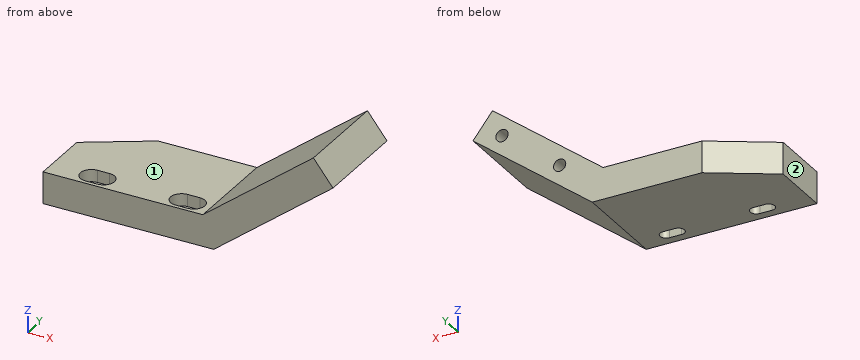
```python
from build123d import *

# Parameters (mm, degrees)
F1_DEPTH = 40
F3_DEPTH = 5
F5_DEPTH = 25
F7_DEPTH = 25
F8_R     = 2.5
F9_DEPTH = 15


with BuildPart() as f1:
    # F0 (on Front) → F1 (new body)
    with BuildSketch(Plane.XZ):
        Polygon((-70, 13), (-70, 0), (0, 0), (48.856667, 38.171011), (40.853068, 48.415151), (-4.476259, 13), align=None)
    extrude(amount=F1_DEPTH)

    # F2 (on face) → F3 (cut)
    with BuildSketch(Plane.XY.offset(13)):
        with BuildLine():
            Line((-16.5, -38.5), (-11.5, -38.5))
            ThreePointArc((-11.5, -38.5), (-7, -34), (-11.5, -29.5))
            Line((-11.5, -29.5), (-16.5, -29.5))
            ThreePointArc((-16.5, -29.5), (-21, -34), (-16.5, -38.5))
        make_face()
        with BuildLine():
            Line((-48.5, -29.5), (-53.5, -29.5))
            ThreePointArc((-53.5, -29.5), (-58, -34), (-53.5, -38.5))
            Line((-53.5, -38.5), (-48.5, -38.5))
            ThreePointArc((-48.5, -38.5), (-44, -34), (-48.5, -29.5))
        make_face()
    extrude(amount=-F3_DEPTH, mode=Mode.SUBTRACT)

    # F4 (on face) → F5 (cut)
    with BuildSketch(Plane.XY.offset(13)):
        with BuildLine():
            Line((-53.5, -36.5), (-48.5, -36.5))
            ThreePointArc((-48.5, -36.5), (-46, -34), (-48.5, -31.5))
            Line((-48.5, -31.5), (-53.5, -31.5))
            ThreePointArc((-53.5, -31.5), (-56, -34), (-53.5, -36.5))
        make_face()
        with BuildLine():
            Line((-11.5, -31.5), (-16.5, -31.5))
            ThreePointArc((-16.5, -31.5), (-19, -34), (-16.5, -36.5))
            Line((-16.5, -36.5), (-11.5, -36.5))
            ThreePointArc((-11.5, -36.5), (-9, -34), (-11.5, -31.5))
        make_face()
    extrude(amount=-F5_DEPTH, mode=Mode.SUBTRACT)

    # F6 (on face) → F7 (cut)
    with BuildSketch(Plane.XY.offset(13)):
        Polygon((-70, 0), (-70, -15), (-45, 0), align=None)
    extrude(amount=-F7_DEPTH, mode=Mode.SUBTRACT)

    # F8 (on face) → F9 (cut)
    with BuildSketch(Plane(origin=(0, 0, 0), x_dir=(-1, 0, 0), z_dir=(0, 1, 0))):
        with Locations((-36.97476, 37.136467)):
            Circle(F8_R)
        with Locations((-13.334437, 18.666622)):
            Circle(F8_R)
    extrude(amount=-F9_DEPTH, mode=Mode.SUBTRACT)


solid = f1.part
```
Geometry: final body of the model. Coordinates: model frame, mm. Face numbers are marked on the shaded views. A direction names the side the tool comes from. Round coordinates to 2 decimals unless told otherwise and drop trailing zeros. Write each loop counter-clockwise with the first axis right and the second up, starting at its lowest first coordinate (ties: lowest second). Pieces come first, ordered by that corner, then holes. Notation, with made-up numbers: (-29.75, 28) -> (-25.75, 28) arc R6 cw to (-25.75, 37) -> close; hole circle Ø10 at (74.5, 42). An arc over 180 degrees is marked (long way). Return JSON: item names as keys, results as strings.
Q1. Section A-A on y = -34. Return the cut outline in (x, z).
From the geometry:
{"outline": "(-70, 0) -> (-56, 0) -> (-56, 8) -> (-58, 8) -> (-58, 13) -> (-70, 13) -> close; (-46, 0) -> (-19, 0) -> (-19, 8) -> (-21, 8) -> (-21, 13) -> (-44, 13) -> (-44, 8) -> (-46, 8) -> close; (-9, 0) -> (0, 0) -> (48.86, 38.17) -> (40.85, 48.42) -> (-4.48, 13) -> (-7, 13) -> (-7, 8) -> (-9, 8) -> close"}
Q2. Ray query, line 1 (Z direction, x = -51, y = -23); line 2 (Y direction, x = -14, z = 5.5); line 3 (X direction, y = -10, z = 18). Return the intervals inside material, ascending.
From the geometry:
{"line 1": "0 to 13", "line 2": "-40 to -36.5, -31.5 to 0", "line 3": "1.92 to 10.92, 15.74 to 23.04"}
Q3. Section D-D on z = 30. Return the cut outline in (x, y), and give its area (3 significant figures).
From the geometry:
{"outline": "(17.28, -40) -> (38.4, -40) -> (38.4, 0) -> (17.28, 0) -> close", "area": "845 mm2"}
Q4. Set-up query: the marked faces 1 and 2. Return all of +Z, -Z, +X, -X, +Y, -Y with unobstructed straight access to the full face (end or side cutting, diameter ignored); none if empty.
From the geometry:
{"face 1": "+Z, -X, +Y, -Y", "face 2": "+Z, -Z, -X, +Y, -Y"}
Q5. Section B-B on y = -10.5. Return the cut outline in (x, z).
From the geometry:
{"outline": "(-62.5, 0) -> (0, 0) -> (48.86, 38.17) -> (40.85, 48.42) -> (-4.48, 13) -> (-62.5, 13) -> close; hole circle Ø5 at (13.33, 18.67); hole circle Ø5 at (36.97, 37.14)"}
Q6. First-contact query: pin 1 Ø4.5 at (x, y) = (-11.5, -32.5) entering from +Z; pin 2 Ø2.5 at (x, z) = (13.5, 18.5) entering from +Y; pin 3 Ø3 at (y, z) = (-25.5, 28.5) entering from +X. Flat tips, straight axial feed; report the tip coordinate or a pass-through.
From the geometry:
{"pin 1": "z = 8", "pin 2": "y = -15", "pin 3": "x = 38.4"}
Q7. Section C-C on x = -59.5. Return the cut outline in (y, z).
From the geometry:
{"outline": "(-40, 0) -> (-8.7, 0) -> (-8.7, 13) -> (-40, 13) -> close"}
